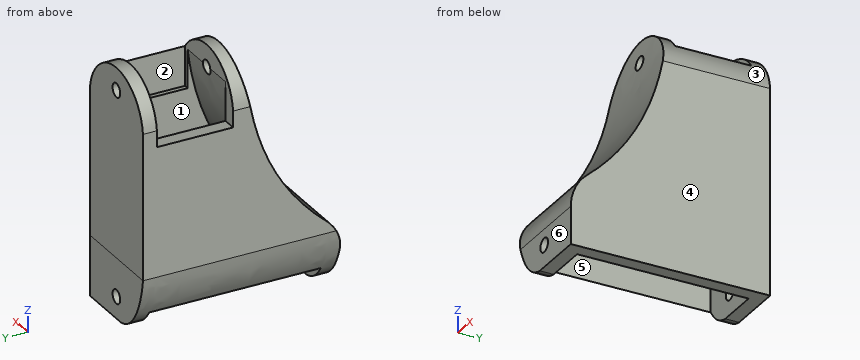
from build123d import *

# Parameters (mm, degrees)
BOSS_EXTRUDE1_DEPTH      = 12
BOSS_EXTRUDE1_DEPTH_BACK = 1
SKETCH1_W                = 20.922356035
SKETCH1_H                = 43
SKETCH14_W               = 14.922356035
SKETCH14_H               = 37
CUT_EXTRUDE6_DEPTH       = 13
SKETCH15_R               = 1.5
CUT_EXTRUDE10_DEPTH      = 43
LOFT8_START              = -19.945599133
LOFT8_DEPTH              = 20.922356013
CUT_EXTRUDE20_DEPTH      = 43
SKETCH22_W               = 16
SKETCH22_H               = 16.433534057
CUT_EXTRUDE21_DEPTH      = 19
CUT_LOFT2_START          = -16.94559915
CUT_LOFT2_DEPTH          = 14.922356033
SKETCH23_R               = 1.5
CUT_EXTRUDE23_DEPTH      = 33
FILLET1_R                = 10


# Read off the part's stored shape, not the designer's step: Loft8, Cut-Loft2
with BuildPart() as part:
    # Sketch1 → Boss-Extrude1 (new, two sides: drawn at the far end of the back side and taken through both)
    with BuildSketch(Plane.XY.offset(-BOSS_EXTRUDE1_DEPTH_BACK)):
        with Locations((-9.484421134, 5.979237668)):
            Rectangle(SKETCH1_W, SKETCH1_H)
    extrude(amount=BOSS_EXTRUDE1_DEPTH + BOSS_EXTRUDE1_DEPTH_BACK)

    # Sketch14 → Cut-Extrude6 (cut)
    with BuildSketch(Plane(origin=(0, 0, -1), x_dir=(-1, 0, 0), z_dir=(0, 0, -1))):
        with Locations((9.484421134, 5.979237668)):
            Rectangle(SKETCH14_W, SKETCH14_H)
    extrude(amount=-CUT_EXTRUDE6_DEPTH, mode=Mode.SUBTRACT)

    # Sketch15 → Cut-Extrude10 (cut)
    with BuildSketch(Plane.XZ.offset(15.520762332)):
        with Locations(Location((-9.484421134, 3.6905228, 0), (0, 0, 270))):
            Circle(SKETCH15_R)
        with BuildLine():
            add(Edge.make_bspline(
                [(-9.484421134, -1), (-16.426209899, -1.809910236), (-19.358305998, 6.878284344), (-19.945599152, 12)],
                knots=[0, 0, 0, 0, 1, 1, 1, 1], degree=3))
            add(Edge.make_bspline(
                [(-19.945599152, 12), (-50.062585738, -15.871811338), (-9.484421134, -1)],
                knots=[0, 0, 0, 1, 1, 1], degree=2))
        make_face()
    extrude(amount=-CUT_EXTRUDE10_DEPTH, mode=Mode.SUBTRACT)

    # Loft8 outline → Loft8 (add)
    with BuildSketch(Plane.YZ.offset(LOFT8_START)):
        with BuildLine():
            add(Edge.make_bspline(
                [(-15.520762333, 12.000000001), (-2.214111033, 21.392948337), (4.785888967, 35.338065027), (5.479237667, 53.835350068)],
                knots=[0, 0, 0, 0, 1, 1, 1, 1], degree=3))
            Line((-15.520762333, 12.000000001), (-12.520762334, 12))
            Line((-12.520762334, 12), (24.479237668, 12.000000002))
            Line((24.479237668, 12.000000002), (27.479237669, 12))
            Line((27.479237669, 12), (27.479237666, 53.835350069))
            Line((27.479237666, 53.835350069), (5.479237667, 53.835350068))
        make_face()
    extrude(amount=LOFT8_DEPTH)

    # Sketch21 → Cut-Extrude20 (cut)
    with BuildSketch(Plane(origin=(0, 27.479237668, 0), x_dir=(1, 0, 0), z_dir=(0, 1, 0))):
        with BuildLine():
            ThreePointArc((-19.945599152, -41.186866189), (-9.484421134, -52.821930397), (0.976756883, -41.186866189))
            add(Edge.make_bspline(
                [(0.976756883, -41.186866189), (22.088375755, -54.528516897), (-10.313654941, -86.662148681), (-35.550608102, -49.144456459), (-19.945599152, -41.186866189)],
                knots=[0, 0, 0, 0, 0.529728329, 1, 1, 1, 1], degree=3))
        make_face()
    extrude(amount=-CUT_EXTRUDE20_DEPTH, mode=Mode.SUBTRACT)

    # Sketch22 → Cut-Extrude21 (cut)
    with BuildSketch(Plane.ZY.offset(19.94559914)):
        with Locations((47.901671706, 16.262470629)):
            Rectangle(SKETCH22_W, SKETCH22_H)
    extrude(amount=-CUT_EXTRUDE21_DEPTH, mode=Mode.SUBTRACT)

    # Cut-Loft2 outline → Cut-Loft2 (cut)
    with BuildSketch(Plane.YZ.offset(CUT_LOFT2_START)):
        with BuildLine():
            add(Edge.make_bspline(
                [(-12.520762331, 12), (-0.657436898, 20.210774423), (6.198051749, 32.307850958), (8.045703611, 48.291229604)],
                knots=[0, 0, 0, 0, 0.898841703, 0.898841703, 0.898841703, 0.898841703], degree=3))
            Line((-12.520762331, 12), (24.47923767, 12))
            Line((24.47923767, 12), (24.47923767, 39.901671701))
            Line((24.47923767, 39.901671701), (8.045703601, 39.901671701))
            Line((8.045703601, 39.901671701), (8.045703611, 48.291229604))
        make_face()
    extrude(amount=CUT_LOFT2_DEPTH, mode=Mode.SUBTRACT)

    # Sketch23 → Cut-Extrude23 (cut)
    with BuildSketch(Plane(origin=(0, 27.479237668, 0), x_dir=(1, 0, 0), z_dir=(0, 1, 0))):
        with Locations(Location((-9.484421063, -47.965150337, 0), (0, 0, 270))):
            Circle(SKETCH23_R)
    extrude(amount=-CUT_EXTRUDE23_DEPTH, mode=Mode.SUBTRACT)

    # Fillet1
    fillet1_edges = [part.edges().sort_by_distance(p)[0] for p in [
        (-9.484421134, -15.520762332, 12),
    ]]
    fillet(fillet1_edges, radius=FILLET1_R)


solid = part.part
Read the model definition and answer for the solid it produces. Units are mm, in the model's axes. Face numbers are marked on the shaded views. A direction names the side the tool comes from. Give positions to 0.01 mm unless a question says otherwise; leave off trailing zeros. Write each question's results on one line, items separated by ' | '.
1. The mould has two halves that part along Y. Classify the marked faces 4, 5 and 6: pulls with the +Y half, pulls with the -Y half, needs draft (parallel to the pull), parting line crosses it, or undercut.
Values:
face 4: needs draft | face 5: undercut | face 6: pulls with the -Y half
2. A tool of negligible diameter and unlimited length cuts with its end or side. For the marked faces 1, 2 and 3, from which of +Z, -Z, +X, -X, +Y, -Y can it reach the whole face along a straight path? Write none if from no direction.
Values:
face 1: -Z | face 2: +Z, -X | face 3: +Z, +Y, -Y
3. Straight lines are drawn through the part: line 1 (X direction, y = 8.5, z = 34); line 2 (Y direction, x = -10.25, z = 18.5); line 3 (Y direction, x = -8.25, z = 32). For each, find the intervals that lie inside material, in ascending order. Write a range as [from, to].
Values:
line 1: x = [-19.95, -16.95], [-2.02, 0.98] | line 2: y = [-7.99, -4.92], [24.48, 27.48] | line 3: y = [0.87, 3.88], [24.48, 27.48]
4. Given pin 1 (6 mm diameter, centred on y = 6.5, z = 6.5, fed in from -X); pin 2 (0.5 mm diameter, centred on x = -1.5, y = 17, fed in from +Z); pin 3 (3.5 mm diameter, centred on x = -9.48, z = 3.69, fed in from +Y); pin 4 (2.5 mm diameter, centred on x = -9.48, z = 47.97, fed in from -Y), each flat-ended and moving along its own axis, determine where each tip first touches the part or whether it passes through.
Values:
pin 1: stops at x = -19.52 | pin 2: stops at z = 39.9 | pin 3: stops at y = 27.48 | pin 4: passes through
